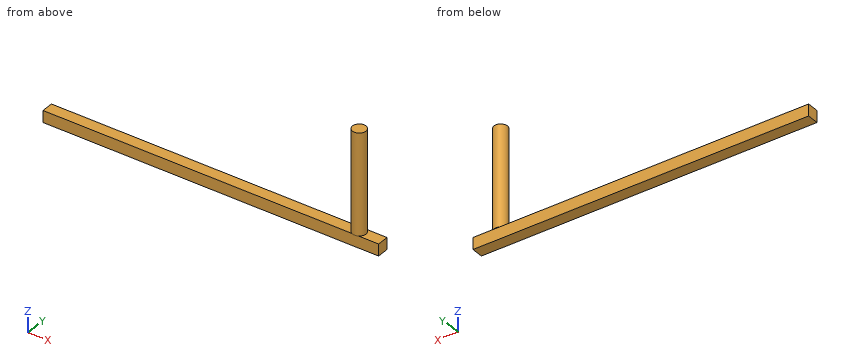
from build123d import *

# Parameters (mm, degrees)
F0_W     = 1000
F0_H     = 35
F1_DEPTH = 35
F2_R     = 20
F3_DEPTH = 300


with BuildPart() as f1:
    # F0 (on Front) → F1 (new body)
    with BuildSketch(Plane.XZ):
        with Locations((-500, 17.5)):
            Rectangle(F0_W, F0_H)
    extrude(amount=-F1_DEPTH)

    # F2 (on face) → F3 (join)
    with BuildSketch(Plane.XY.offset(35)):
        with Locations((-70, 17.5)):
            Circle(F2_R)
    extrude(amount=F3_DEPTH)


solid = f1.part
Can you work these out from the model? Positions are in its coordinate system, mm. Coordinates: 2 decimals unless noted, no trailing zeros. Loops run counter-clockwise (first coordinate to the right, second up) from the corner with the lowest first, then second, coordinate; pieces in that order, holes last. Notation, with made-up numbers: (85, 18.25) - (104, 18.25) arc R37 ccw to (104, 55.25) - close; hole circle Ø1 at (42.25, 60). An arc over 180 degrees is marked (long way). Put each result on its own line as item: value. Start each with the question number.
Item 1: Suppose I cut it at C-C (z = 197.5). Please give me the cut outline in (x, y).
Item 2: Suppose I cut it at B-B (x = -300.5). Please give me the cut outline in (y, z).
Item 3: Suppose I cut it at A-A (y = 17.5). Please give me the cut outline in (x, z).
Item 4: For pin 1 (6 mm diameter, centred on x = -101, y = 4.5, fed in from +Z); pin 2 (0.8 mm diameter, centred on x = -72, y = -2, fed in from -Z); pin 3 (5 mm diameter, centred on y = 13, z = 282.5, fed in from -X), each with a flat end and sliding along its axis, tell me the tip position at first contact or that it passes through.
Item 5: If I drill on line 1 along Z through (x, y) = (-663.5, 20.5); line 2 along X through (y, z) = (19, 145), over which ranges is the centre line in solid material (lowest first)?
Here are the results:
1. outline: circle Ø40 at (-70, 17.5)
2. outline: (0, 0) - (35, 0) - (35, 35) - (0, 35) - close
3. outline: (-1000, 0) - (0, 0) - (0, 35) - (-50, 35) - (-50, 335) - (-90, 335) - (-90, 35) - (-1000, 35) - close
4. pin 1: z = 35
4. pin 2: z = 35
4. pin 3: x = -89.9
5. line 1: 0 to 35
5. line 2: -89.94 to -50.06
